from build123d import *

# Parameters (mm, degrees)
F2_R    = 0.508
F3_R    = 0.508
F4_SIZE = 0.254


with BuildPart() as f1:
    # F0 (on Front) → F1 (revolve)
    with BuildSketch(Plane.XZ):
        with BuildLine():
            Line((-12.7, 0), (0, 0))
            ThreePointArc((0, 0), (-1.872948, 2.941347), (-5.323115, 2.435581))
            Line((-5.323115, 2.435581), (-5.323115, 2.027367))
            Line((-5.323115, 2.027367), (-7.920302, 2.027367))
            Line((-7.920302, 2.027367), (-7.920302, 2.435581))
            Line((-7.920302, 2.435581), (-7.920302, 3.882198))
            Line((-7.920302, 3.882198), (-8.555302, 3.882198))
            Line((-8.555302, 3.882198), (-8.995197, 5.073581))
            Line((-8.995197, 5.073581), (-9.525, 3.919367))
            Line((-9.525, 3.919367), (-10.16, 3.919367))
            Line((-10.16, 3.919367), (-10.16, 6.35))
            Line((-10.16, 6.35), (-12.7, 6.35))
            Line((-12.7, 6.35), (-12.7, 0))
        make_face()
    revolve(axis=Axis((-6.35, 0, 0), (-1, 0, 0)))

    # F2
    f2_edges = [f1.edges().sort_by_distance(p)[0] for p in [
        (-5.323115, 0, -2.435581),
    ]]
    fillet(f2_edges, radius=F2_R)

    # F3
    f3_edges = [f1.edges().sort_by_distance(p)[0] for p in [
        (-10.16, 0, -6.35),
    ]]
    fillet(f3_edges, radius=F3_R)

    # F4
    f4_edges = [f1.edges().sort_by_distance(p)[0] for p in [
        (-7.920302, 0, -3.882198),
    ]]
    chamfer(f4_edges, length=F4_SIZE)


solid = f1.part
Verification items for the finished model (mm, model axes). A direction names the side the tool comes from. Round coordinates to 2 decimals unless told otherwise and drop trailing zeros. Order: outer loops, then holes, each group sorted by start corner. A loop starts at its lowest first (then second) coordinate and runs counter-clockwise, first axis right, second up.
1. Thickness scan on L1, parallel to X at y = -3.75, z = 3; L2, parallel to X at y = -0.5, z = 5.5; L3, parallel to Y at x = -11.5, z = 2. Record the ranges inside material, lowest first.
Final values:
L1: x = -12.7 to -10.16, -9.12 to -8.9
L2: x = -12.7 to -10.16
L3: y = -6.03 to 6.03
2. Access from +Z, -Z, +X, -X, +Y, -Y to the whole of each face (thin tool, end or side, straight path). Record for faces 1 (the cylindrical face through (-8.37, 3.85, -0.51)), 2 (the flat face through (-10.16, -4, -1)).
Final values:
face 1: +X
face 2: none
3. Section check B-B on x = -7.25. Record the cut outline in (y, z), then the cut area to 3 significant figures.
Final values:
outline: circle Ø4.05 at (0, 0)
area: 12.9 mm2
4. Release check for a two-part mould opening along X. For faces 3 (the cylindrical face through (-11.7, -6.2, -1.38)), 4 (the cylindrical face through (-6.64, 0.609, 1.934)), 5 (the flat face through (-12.7, 0, 0)) record: +X half, -X half, draft (parallel to the pull), parting line (faces both ways), or undercut.
Final values:
face 3: draft
face 4: undercut
face 5: -X half
5. Section check A-A on x = -11.25. Record the cut outline in (y, z).
Final values:
outline: circle Ø12.7 at (0, 0)
6. Go/stop test with flat-tipped pins: P1, Ø6, axis at y = -1.5, z = -1.5, coming from the +X side; P2, Ø4, axis at x = -5, y = -1, coming from the -Z side; P3, Ø4, axis at x = -8.5, y = -2, coming from the +Z side; P4, Ø1, axis at x = -11, z = -4.5, coming from the +Y side. Record where each tip stops, or that it passes through.
Final values:
P1: stops at x = 0
P2: stops at z = -3.23
P3: stops at z = 6.12
P4: stops at y = 4.93
